Answer from the drawing. Dimensions are ordinates in mm from the lowest x, y and z of the part. Coordinates: 2 decimals unless noted, no trailing zeros. Write each loop counter-clockwise with the first axis right and the second up, starting at its lowest first coordinate (ties: lowest second). Pieces come first, ordered by that corner, then holes. Notation, with made-up numbers: (13, 13.25) -> (42, 13.25) arc R7 ccw to (42, 19.25) -> close; hole circle Ø10 at (-18.75, -22.5). An arc over 180 degrees is marked (long way). Use CSV: the item, a comma, the result in double quotes.
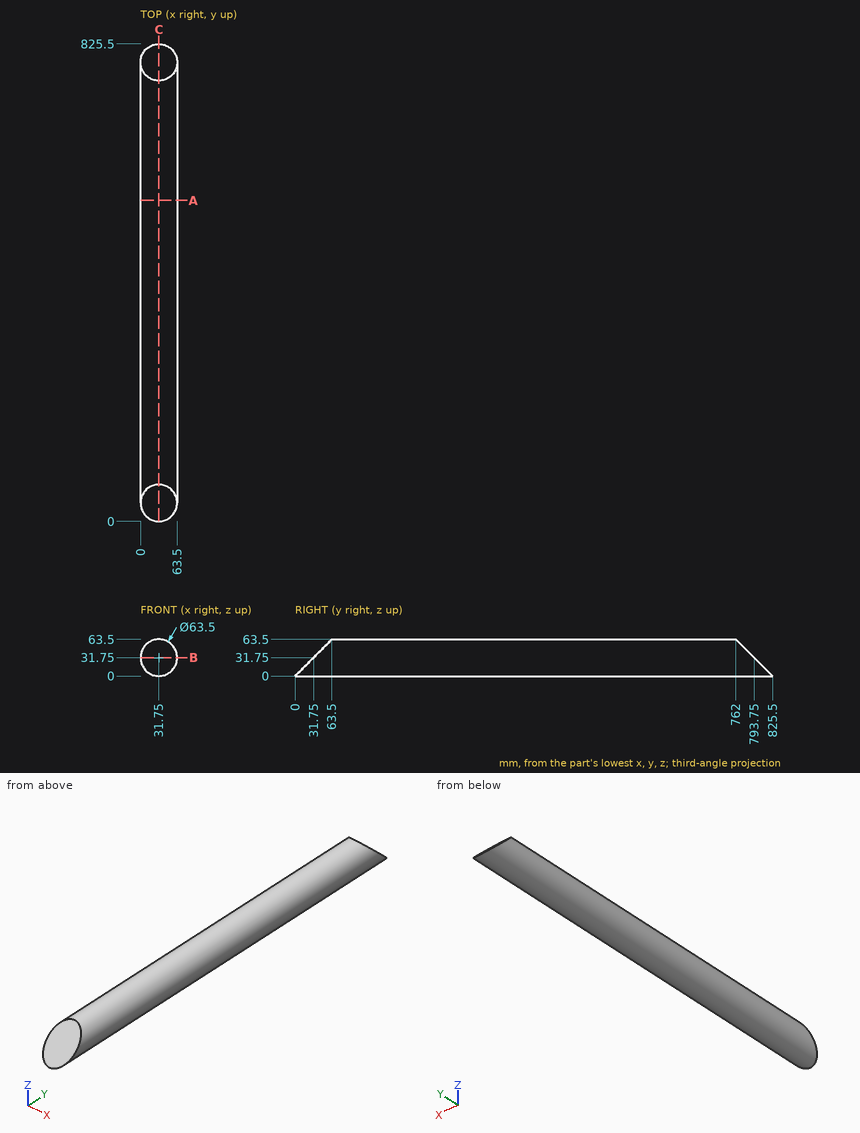
1. Find the intervals of material crossed by line 1 along Z through (x, y) = (29, 737.5); line 2 along Z through (x, y) = (31, 132.5); line 3 along Y through (x, z) = (6, 23.5), in increasing order.
Solutions:
line 1,"z = 0.12 to 63.38"
line 2,"z = 0.01 to 63.49"
line 3,"y = 23.5 to 802"
2. Each of these flat-tipped pins is pushed along its axis until it touches: pin 1 Ø1.5 at (x, y) = (7, 286.5) entering from -Z; pin 2 Ø4 at (x, y) = (53, 159) entering from +Z; pin 3 Ø3 at (x, z) = (21.5, 30) entering from -Y. Where does it stop, or does it pass through?
Solutions:
pin 1,"stops at z = 10.96"
pin 2,"stops at z = 57"
pin 3,"stops at y = 28.5"
3. A cutting plane is placed at A-A (y = 555). Give the vertices of the cut face in (x, z), and give its area (3 significant figures).
Solutions:
outline,"circle Ø63.5 at (31.75, 31.75)"
area,"3,170 mm^2"
4. A cutting plane is placed at C-C (x = 31.75). Give the vertices of the cut face in (y, z), and give its area (3 significant figures).
Solutions:
outline,"(0, 0) -> (825.5, 0) -> (762, 63.5) -> (63.5, 63.5) -> close"
area,"48,400 mm^2"
5. A cutting plane is placed at B-B (z = 31.75). Give the vertices of the cut face in (x, y).
Solutions:
outline,"(0, 31.75) -> (63.5, 31.75) -> (63.5, 793.75) -> (0, 793.75) -> close"
